Check sheet for the modelled part. Datum: model origin and axes. Units: mm. A direction names the side the tool comes from. Round coordinates to 2 decimals unless told otherwise and drop trailing zeros. Write each loop counter-clockwise with the first axis right and the second up, starting at its lowest first coordinate (ties: lowest second). Pieces come first, ordered by that corner, then holes.
from build123d import *

# Parameters (mm, degrees)
SKETCH_1_R            = 55
EXTRUDE_1_DEPTH       = 5
SKETCH_2_R            = 49.9
EXTRUDE_2_DEPTH       = 5
SKETCH_3_W            = 35
SKETCH_3_H            = 45
EXTRUDE_3_DEPTH       = 25
SKETCH_4_W            = 20.2
SKETCH_4_H            = 10.3
CUT_EXTRUDE_1_DEPTH   = 78.5
SKETCH_5_R            = 4.1
CUT_EXTRUDE_2_DEPTH   = 11
SKETCH_6_R            = 2.75
CUT_EXTRUDE_3_DEPTH   = 36
CHAMFER1_SIZE         = 2
CHAMFER1_SIZE2        = 0.535898385
CHAMFER1_PART_2_SIZE  = 2
CHAMFER1_PART_2_SIZE2 = 0.535898385
CHAMFER1_PART_3_SIZE  = 2
CHAMFER1_PART_3_SIZE2 = 0.535898385
CHAMFER1_PART_4_SIZE  = 2
CHAMFER1_PART_4_SIZE2 = 0.535898385
SKETCH2_W             = 35.065209797
SKETCH2_H             = 45
CUT_EXTRUDE1_DEPTH    = 12.5
BOSS_EXTRUDE1_START   = -2
SKETCH4_W             = 70
SKETCH4_H             = 45
BOSS_EXTRUDE1_DEPTH   = 5.35
SKETCH5_R             = 4.15
CUT_EXTRUDE2_DEPTH    = 16.3500001
CUT_EXTRUDE3_DEPTH    = 6.5
SKETCH7_W             = 20
SKETCH7_H             = 34
CUT_EXTRUDE4_DEPTH    = 5
CHAMFER2_SIZE         = 1
CHAMFER2_SIZE2        = 2.747477419
SKETCH8_W             = 12.8
SKETCH8_H             = 15
CUT_EXTRUDE5_DEPTH    = 11.0000001
SKETCH9_W             = 10
SKETCH9_H             = 15
CUT_EXTRUDE6_DEPTH    = 4.2


with BuildPart() as part:
    # Эскиз1 → Бобышка-Вытянуть1 (new body)
    with BuildSketch(Plane(origin=(0, 0, 0), x_dir=(1, 0, 0), z_dir=(0, 1, 0))):
        Circle(SKETCH_1_R)
    extrude(amount=EXTRUDE_1_DEPTH)

    # Эскиз2 → Бобышка-Вытянуть2 (add)
    with BuildSketch(Plane(origin=(0, 5, 0), x_dir=(1, 0, 0), z_dir=(0, 1, 0))):
        Circle(SKETCH_2_R)
    extrude(amount=EXTRUDE_2_DEPTH)

    # Эскиз3 → Бобышка-Вытянуть3 (add)
    with BuildSketch(Plane.XZ):
        Rectangle(SKETCH_3_W, SKETCH_3_H)
    extrude(amount=EXTRUDE_3_DEPTH)

    # Эскиз4 → Вырез-Вытянуть1 (cut, through all)
    with BuildSketch(Plane.XY.offset(22.5)):
        with Locations((0, -12.5)):
            Rectangle(SKETCH_4_W, SKETCH_4_H)
    extrude(amount=-CUT_EXTRUDE_1_DEPTH, mode=Mode.SUBTRACT)

    # Эскиз5 → Вырез-Вытянуть2 (cut, through all)
    with BuildSketch(Plane.XZ):
        with Locations((33.592198598, -32.871936263)):
            Circle(SKETCH_5_R)
        with Locations((-33.591727056, -32.872418125)):
            Circle(SKETCH_5_R)
        with Locations((-33.591727056, 32.872418125)):
            Circle(SKETCH_5_R)
        with Locations((33.483215177, 32.983215177)):
            Circle(SKETCH_5_R)
    extrude(amount=-CUT_EXTRUDE_2_DEPTH, mode=Mode.SUBTRACT)

    # Эскиз6 → Вырез-Вытянуть3 (cut, through all)
    with BuildSketch(Plane(origin=(0, 10, 0), x_dir=(1, 0, 0), z_dir=(0, 1, 0))):
        with Locations((-17.999799176, 27.999999999)):
            Circle(SKETCH_6_R)
    extrude(amount=-CUT_EXTRUDE_3_DEPTH, mode=Mode.SUBTRACT)

    # Chamfer1
    chamfer1_edges = [part.edges().sort_by_distance(p)[0] for p in [
        (0.000357897, 10, -49.899999999),
    ]]
    chamfer1_side = [part.faces().sort_by_distance(p)[0] for p in [
        (0.000357897, 7.5, -49.899999999),
    ]]
    chamfer(chamfer1_edges, length=CHAMFER1_SIZE, length2=CHAMFER1_SIZE2, reference=chamfer1_side[0])

    # Chamfer1 part 2
    chamfer1_part_2_edges = [part.edges().sort_by_distance(p)[0] for p in [
        (-49.9, 10, 0),
    ]]
    chamfer1_part_2_side = [part.faces().sort_by_distance(p)[0] for p in [
        (-49.9, 7.5, 0),
    ]]
    chamfer(chamfer1_part_2_edges, length=CHAMFER1_PART_2_SIZE, length2=CHAMFER1_PART_2_SIZE2, reference=chamfer1_part_2_side[0])

    # Chamfer1 part 3
    chamfer1_part_3_edges = [part.edges().sort_by_distance(p)[0] for p in [
        (-0.08242255, 10, 49.899931929),
    ]]
    chamfer1_part_3_side = [part.faces().sort_by_distance(p)[0] for p in [
        (-0.08242255, 7.5, 49.899931929),
    ]]
    chamfer(chamfer1_part_3_edges, length=CHAMFER1_PART_3_SIZE, length2=CHAMFER1_PART_3_SIZE2, reference=chamfer1_part_3_side[0])

    # Chamfer1 part 4
    chamfer1_part_4_edges = [part.edges().sort_by_distance(p)[0] for p in [
        (49.899931657, 10, 0.082587101),
    ]]
    chamfer1_part_4_side = [part.faces().sort_by_distance(p)[0] for p in [
        (49.899931657, 7.5, 0.082587101),
    ]]
    chamfer(chamfer1_part_4_edges, length=CHAMFER1_PART_4_SIZE, length2=CHAMFER1_PART_4_SIZE2, reference=chamfer1_part_4_side[0])

    # Sketch2 → Cut-Extrude1 (cut)
    with BuildSketch(Plane.XZ.offset(25)):
        with Locations((-0.032604899, 0)):
            Rectangle(SKETCH2_W, SKETCH2_H)
    extrude(amount=-CUT_EXTRUDE1_DEPTH, mode=Mode.SUBTRACT)

    # Sketch4 → Boss-Extrude1 (add)
    with BuildSketch(Plane.XZ.offset(7.35).offset(BOSS_EXTRUDE1_START)):
        Rectangle(SKETCH4_W, SKETCH4_H)
    extrude(amount=-BOSS_EXTRUDE1_DEPTH)

    # Sketch5 → Cut-Extrude2 (cut, through all)
    with BuildSketch(Plane.XZ.offset(5.35)):
        with Locations((25, 15)):
            Circle(SKETCH5_R)
        with Locations((-25, 15)):
            Circle(SKETCH5_R)
        with Locations((25, -15)):
            Circle(SKETCH5_R)
        with Locations((-25, -15)):
            Circle(SKETCH5_R)
    extrude(amount=-CUT_EXTRUDE2_DEPTH, mode=Mode.SUBTRACT)

    # Sketch6 → Cut-Extrude3 (cut)
    with BuildSketch(Plane(origin=(0, 10, 0), x_dir=(1, 0, 0), z_dir=(0, 1, 0))):
        Polygon((-18.504809472, -11.25), (-25, -7.5), (-31.495190528, -11.25), (-31.495190528, -18.75), (-25, -22.5), (-18.504809472, -18.75), align=None)
        Polygon((31.495190528, -11.25), (25, -7.5), (18.504809472, -11.25), (18.504809472, -18.75), (25, -22.5), (31.495190528, -18.75), align=None)
        Polygon((31.495190528, 18.75), (25, 22.5), (18.504809472, 18.75), (18.504809472, 11.25), (25, 7.5), (31.495190528, 11.25), align=None)
        Polygon((-18.504809472, 18.75), (-25, 22.5), (-31.495190528, 18.75), (-31.495190528, 11.25), (-25, 7.5), (-18.504809472, 11.25), align=None)
    extrude(amount=-CUT_EXTRUDE3_DEPTH, mode=Mode.SUBTRACT)

    # Sketch7 → Cut-Extrude4 (cut)
    with BuildSketch(Plane(origin=(0, 10, 0), x_dir=(1, 0, 0), z_dir=(0, 1, 0))):
        Rectangle(SKETCH7_W, SKETCH7_H)
    extrude(amount=-CUT_EXTRUDE4_DEPTH, mode=Mode.SUBTRACT)

    # Chamfer2
    chamfer2_edges = [part.edges().sort_by_distance(p)[0] for p in [
        (-18.504809472, 10, 15),
        (-21.752404736, 10, 9.375),
        (-28.247595264, 10, 9.375),
        (-31.495190528, 10, 15),
        (-28.247595264, 10, 20.625),
        (-21.752404736, 10, 20.625),
        (31.495190528, 10, 15),
        (28.247595264, 10, 9.375),
        (21.752404736, 10, 9.375),
        (18.504809472, 10, 15),
        (21.752404736, 10, 20.625),
        (28.247595264, 10, 20.625),
        (31.495190528, 10, -15),
        (28.247595264, 10, -20.625),
        (21.752404736, 10, -20.625),
        (18.504809472, 10, -15),
        (21.752404736, 10, -9.375),
        (28.247595264, 10, -9.375),
        (-18.504809472, 10, -15),
        (-21.752404736, 10, -20.625),
        (-28.247595264, 10, -20.625),
        (-31.495190528, 10, -15),
        (-28.247595264, 10, -9.375),
        (-21.752404736, 10, -9.375),
    ]]
    chamfer2_side = [part.faces().sort_by_distance(p)[0] for p in [
        (29.567670169, 10, 29.126140435),
    ]]
    chamfer(chamfer2_edges, length=CHAMFER2_SIZE, length2=CHAMFER2_SIZE2, reference=chamfer2_side[0])

    # Sketch8 → Cut-Extrude5 (cut, through all)
    with BuildSketch(Plane.XZ):
        with Locations((-19, -32)):
            Rectangle(SKETCH8_W, SKETCH8_H)
    extrude(amount=-CUT_EXTRUDE5_DEPTH, mode=Mode.SUBTRACT)

    # Sketch9 → Cut-Extrude6 (cut)
    with BuildSketch(Plane(origin=(0, 10, 0), x_dir=(1, 0, 0), z_dir=(0, 1, 0))):
        with Locations((-7.6, 32)):
            Rectangle(SKETCH9_W, SKETCH9_H)
    extrude(amount=-CUT_EXTRUDE6_DEPTH, mode=Mode.SUBTRACT)


solid = part.part
1. Sectioned sample at A-A, the plane y = -9.75. Enter the section's corners in (x, z).
2. Sectioned sample at B-B, the plane y = -1.5. Enter the section's corners in (x, z), plus the area to 3 significant figures.
3. Sectioned sample at C-C, the plane z = 0. Enter the section's corners in (x, y), plus the area to 3 significant figures.
4. Release check for a two-part mould opening along Z. For faces 3 (the cylindrical face through (-49.898, 6.479, -0.499)), 4 (the flat face through (-31.495, 5, -15)), 5 (the flat face through (17.5, -9, 0)) record: released by +Z, released by -Z, zero draft, split by the parting line, or undercut.
5. Sectioned sample at D-D, the plane x = -27. Give the number of separate pieces and of enclosed holes in the cut face, plus the area to 3 significant figures.
6. Go/stop test with flat-tipped pins: pin 1 (6 mm diameter, centred on x = 10, y = -7, fed in from -Z); pin 2 (4 mm diameter, centred on y = 7.5, z = -15, fed in from -X); pin 3 (4.5 mm diameter, centred on y = -3, z = -1.5, fed in from +X); pin 4 (10.5 mm diameter, centred on x = 25.5, z = 11.5, fed in from +Y). Record where each tip stops, or that it passes through.
7. Scan lines: line 1 along X through (y, z) = (7, -8); line 2 along X through (y, z) = (1, 31); line 3 along Z through (x, y) = (-26, 3). Record each from-to range of solid material in increasing order.
8. Set-up check for faces 1 (the cylindrical face through (-25.9, -0.99, 10.95)), 2 (the flat face through (-28.29, 5.4, 20.6)): record each of +Z, -Z, +X, -X, +Y, -Y from which the full face is reachable in a straight line by a thin tool's end or side.
Computed values:
1. outline: (-17.5, -22.5) - (-10.1, -22.5) - (-10.1, 22.5) - (-17.5, 22.5) - close; (10.1, -22.5) - (17.5, -22.5) - (17.5, 22.5) - (10.1, 22.5) - close
2. outline: (-35, -22.5) - (35, -22.5) - (35, 22.5) - (-35, 22.5) - close; hole circle Ø8.3 at (-25, -15); hole circle Ø8.3 at (-25, 15); hole circle Ø8.3 at (25, -15); hole circle Ø8.3 at (25, 15)
2. area: 2,930 mm2
3. outline: (-55, 0) - (-35, 0) - (-35, -5.35) - (-17.5, -5.35) - (-17.5, -12.5) - (-10.1, -12.5) - (-10.1, -7.35) - (10.1, -7.35) - (10.1, -12.5) - (17.5, -12.5) - (17.5, -5.35) - (35, -5.35) - (35, 0) - (55, 0) - (55, 5) - (49.9, 5) - (49.9, 8) - (49.36, 10) - (10, 10) - (10, 5) - (-10, 5) - (-10, 10) - (-49.36, 10) - (-49.9, 8) - (-49.9, 5) - (-55, 5) - close
3. area: 1,470 mm2
4. face 3: split by the parting line
4. face 4: undercut
4. face 5: zero draft
5. separate pieces: 3
5. enclosed holes: 0
5. area: 838 mm2
6. pin 1: stops at z = -22.5
6. pin 2: stops at x = -48.18
6. pin 3: stops at x = 35
6. pin 4: stops at y = 10
7. line 1: x = -49.25 to -25.87, -24.13 to -10, 10 to 24.13, 25.87 to 49.25
7. line 2: x = -45.43 to -37.24, -29.94 to 29.89, 37.07 to 45.43
7. line 3: z = -48.47 to -19.03, -10.97 to 10.97, 19.03 to 48.47
8. face 1: +Y, -Y
8. face 2: +Y
